Geometry check sheet. Reference: the model listing, model coordinates, mm. A direction names the side the tool comes from. Round coordinates to 2 decimals unless told otherwise and drop trailing zeros. Order: outer loops, then holes, each group sorted by start corner. A loop starts at its lowest first (then second) coordinate and runs counter-clockwise, first axis right, second up. Notation, with made-up numbers: (42.25, 17) -> (94.25, 17) arc R23 cw to (94.25, 54) -> close; hole circle Ø11 at (28, 61.5). An arc over 180 degrees is marked (long way). Use a Markdown table: item, result. Add a question column.
Item 1: Sectioned sample at A-A, the plane z = -24. Record the cut outline in (x, y), and give its area (3 significant figures).
Item 2: Mould release check, pull along Y, two halves, no side actions. Record for faces 1 (the cylindrical face through (93.92, 277.14, -2.39)), 2 (the flat face through (94, -26, -50.8)), 3 (the flat face through (94, -3.038, -24)): pulls with the +Y half, pulls with the -Y half, needs draft (parallel to the pull), parting line crosses it, or undercut.
Item 3: Material ranges on probe 1 along X at (y, z) = (254, 1.05); probe 2 along Y at (x, z) = (165.1, -49.25); probe 3 along Y at (x, z) = (25.4, -49.05), recorded low to high. Write a range as [from, to].
Item 4: Sectioned sample at C-C, the plane y = 211.5. Record the cut outline in (x, z), and give its area (3 significant figures).
Item 5: Set-up check for faces 4 (the flat face through (94, 138, 3.038)), 5 (the flat face through (94, 142, 0)), 6 (the flat face through (97, 306, -47.762)): record each of +Z, -Z, +X, -X, +Y, -Y from which the full face is reachable in a straight line by a thin tool's end or side.
Item 6: Sectioned sample at B-B, the plane x = 146.5. Record the cut outline in (y, z) (1 decimal).
Item 7: Gauge pin test, flat ends, axial feed: pin 1 Ø4 at (x, y) = (27, 137.5) entering from -Z; pin 2 Ø16 at (x, z) = (64.5, -23) entering from -Y; pin 3 Ø15 at (x, y) = (54.5, 308.5) entering from +Z. Record the tip position at first contact, or that the pin passes through.
from build123d import *

# Parameters (mm, degrees)
BASE_FLANGE1_DEPTH           = 190.5
SKETCH3_R                    = 2.778125
CUT_EXTRUDE1_DEPTH           = 3.03784
EDGE_FLANGE1_STRIP_W         = 28.02636
EDGE_FLANGE1_STRIP_H         = 3.03784
EDGE_FLANGE1_STRIP_CUT_DEPTH = 190.5
EDGE_FLANGE1_DEPTH           = 190.5
EDGE_FLANGE2_STRIP_W         = 28.02636
EDGE_FLANGE2_STRIP_H         = 3.03784
EDGE_FLANGE2_STRIP_CUT_DEPTH = 190.5
EDGE_FLANGE2_DEPTH           = 190.5
FILLET1_R                    = 3.175
SKETCH12_R                   = 3.96875
CUT_EXTRUDE2_DEPTH           = 3.03784


# Sheet-metal steps are written as plain solids
with BuildPart() as part:
    # Sketch1 → Base-Flange1 (new body)
    with BuildSketch(Plane(origin=(0, 0, 0), x_dir=(0, 0, -1), z_dir=(1, 0, 0))):
        with BuildLine():
            Line((50.8, 279.4), (7.9375, 279.4))
            ThreePointArc((7.9375, 279.4), (2.324839924, 277.075160076), (0, 271.4625))
            Line((0, 271.4625), (0, 7.9375))
            ThreePointArc((0, 7.9375), (2.324839924, 2.324839924), (7.9375, 0))
            Line((7.9375, 0), (50.8, 0))
            Line((50.8, 0), (50.8, -3.03784))
            Line((50.8, -3.03784), (7.9375, -3.03784))
            ThreePointArc((7.9375, -3.03784), (0.17676266, 0.17676266), (-3.03784, 7.9375))
            Line((-3.03784, 7.9375), (-3.03784, 271.4625))
            ThreePointArc((-3.03784, 271.4625), (0.17676266, 279.22323734), (7.9375, 282.43784))
            Line((7.9375, 282.43784), (50.8, 282.43784))
            Line((50.8, 282.43784), (50.8, 279.4))
        make_face()
    extrude(amount=BASE_FLANGE1_DEPTH)

    # Sketch3 → Cut-Extrude1 (cut)
    with BuildSketch(Plane.XY.offset(3.03784)):
        with Locations((171.45, 254)):
            Circle(SKETCH3_R)
        with Locations((19.05, 254)):
            Circle(SKETCH3_R)
        with Locations((171.45, 25.4)):
            Circle(SKETCH3_R)
        with Locations((19.05, 25.4)):
            Circle(SKETCH3_R)
    extrude(amount=-CUT_EXTRUDE1_DEPTH, mode=Mode.SUBTRACT)

    # Edge-Flange1 strip (across the edge) → Edge-Flange1 strip cut (cut)
    with BuildSketch(Plane(origin=(0, -3.03784, -50.8), x_dir=(0, 0, 1), z_dir=(1, 0, 0))):
        with Locations((-3.03784, -1.51892)):
            Rectangle(EDGE_FLANGE1_STRIP_W, EDGE_FLANGE1_STRIP_H)
    extrude(amount=EDGE_FLANGE1_STRIP_CUT_DEPTH, mode=Mode.SUBTRACT)

    # Edge-Flange1 section (across the edge) → Edge-Flange1 (add)
    with BuildSketch(Plane(origin=(0, -3.03784, -50.8), x_dir=(0, 0, 1), z_dir=(1, 0, 0))):
        with BuildLine():
            Line((0, 7.9375), (0, 38.1))
            Line((0, 38.1), (3.03784, 38.1))
            Line((3.03784, 38.1), (3.03784, 7.9375))
            ThreePointArc((3.03784, 7.9375), (5.362679924, 2.324839924), (10.97534, 0))
            Line((10.97534, 0), (10.97534, -3.03784))
            ThreePointArc((10.97534, -3.03784), (3.21460266, 0.17676266), (0, 7.9375))
        make_face()
    extrude(amount=EDGE_FLANGE1_DEPTH)

    # Edge-Flange2 strip (across the edge) → Edge-Flange2 strip cut (cut)
    with BuildSketch(Plane(origin=(190.5, 282.43784, -50.8), x_dir=(0, 0, 1), z_dir=(-1, 0, 0))):
        with Locations((-3.03784, -1.51892)):
            Rectangle(EDGE_FLANGE2_STRIP_W, EDGE_FLANGE2_STRIP_H)
    extrude(amount=EDGE_FLANGE2_STRIP_CUT_DEPTH, mode=Mode.SUBTRACT)

    # Edge-Flange2 section (across the edge) → Edge-Flange2 (add)
    with BuildSketch(Plane(origin=(190.5, 282.43784, -50.8), x_dir=(0, 0, 1), z_dir=(-1, 0, 0))):
        with BuildLine():
            Line((0, 7.9375), (0, 38.1))
            Line((0, 38.1), (3.03784, 38.1))
            Line((3.03784, 38.1), (3.03784, 7.9375))
            ThreePointArc((3.03784, 7.9375), (5.362679924, 2.324839924), (10.97534, 0))
            Line((10.97534, 0), (10.97534, -3.03784))
            ThreePointArc((10.97534, -3.03784), (3.21460266, 0.17676266), (0, 7.9375))
        make_face()
    extrude(amount=EDGE_FLANGE2_DEPTH)

    # Fillet1
    fillet1_edges = [part.edges().sort_by_distance(p)[0] for p in [
        (190.5, 320.53784, -49.28108),
        (0, 320.53784, -49.28108),
        (0, -41.13784, -49.28108),
        (190.5, -41.13784, -49.28108),
    ]]
    fillet(fillet1_edges, radius=FILLET1_R)

    # Sketch12 → Cut-Extrude2 (cut)
    with BuildSketch(Plane.XY.offset(-47.76216)):
        with Locations((25.4, 304.66284)):
            Circle(SKETCH12_R)
        with Locations((165.1, 304.66284)):
            Circle(SKETCH12_R)
        with Locations((165.1, -25.26284)):
            Circle(SKETCH12_R)
        with Locations((25.4, -25.26284)):
            Circle(SKETCH12_R)
    extrude(amount=-CUT_EXTRUDE2_DEPTH, mode=Mode.SUBTRACT)


solid = part.part
Found:
| question | item | result |
|---|---|---|
| 1 | outline | (0, -3.04) -> (190.5, -3.04) -> (190.5, 0) -> (0, 0) -> close; (0, 279.4) -> (190.5, 279.4) -> (190.5, 282.44) -> (0, 282.44) -> close |
| 1 | area | 1,160 mm2 |
| 2 | face 1 | undercut |
| 2 | face 2 | needs draft |
| 2 | face 3 | pulls with the -Y half |
| 3 | probe 1 | x = [0, 16.27], [21.83, 168.67], [174.23, 190.5] |
| 3 | probe 2 | y = [-41.14, -29.23], [-21.29, -5.35], [284.75, 300.69], [308.63, 320.54] |
| 3 | probe 3 | y = [-41.14, -29.23], [-21.29, -5.03], [284.43, 300.69], [308.63, 320.54] |
| 4 | outline | (0, 0) -> (190.5, 0) -> (190.5, 3.04) -> (0, 3.04) -> close |
| 4 | area | 579 mm2 |
| 5 | face 4 | +Z, +X, -X, +Y, -Y |
| 5 | face 5 | -Z, +X, -X |
| 5 | face 6 | +Z, +X, -X, +Y |
| 6 | outline | (-41.1, -50.8) -> (-11, -50.8) arc R11 ccw to (0, -39.8) -> (0, -7.9) arc R7.9 cw to (7.9, 0) -> (271.5, 0) arc R7.9 cw to (279.4, -7.9) -> (279.4, -39.8) arc R11 ccw to (290.4, -50.8) -> (320.5, -50.8) -> (320.5, -47.8) -> (290.4, -47.8) arc R7.9 cw to (282.4, -39.8) -> (282.4, -7.9) arc R11 ccw to (271.5, 3) -> (7.9, 3) arc R11 ccw to (-3, -7.9) -> (-3, -39.8) arc R7.9 cw to (-11, -47.8) -> (-41.1, -47.8) -> close |
| 7 | pin 1 | stops at z = 0 |
| 7 | pin 2 | stops at y = -3.04 |
| 7 | pin 3 | stops at z = -47.76 |
